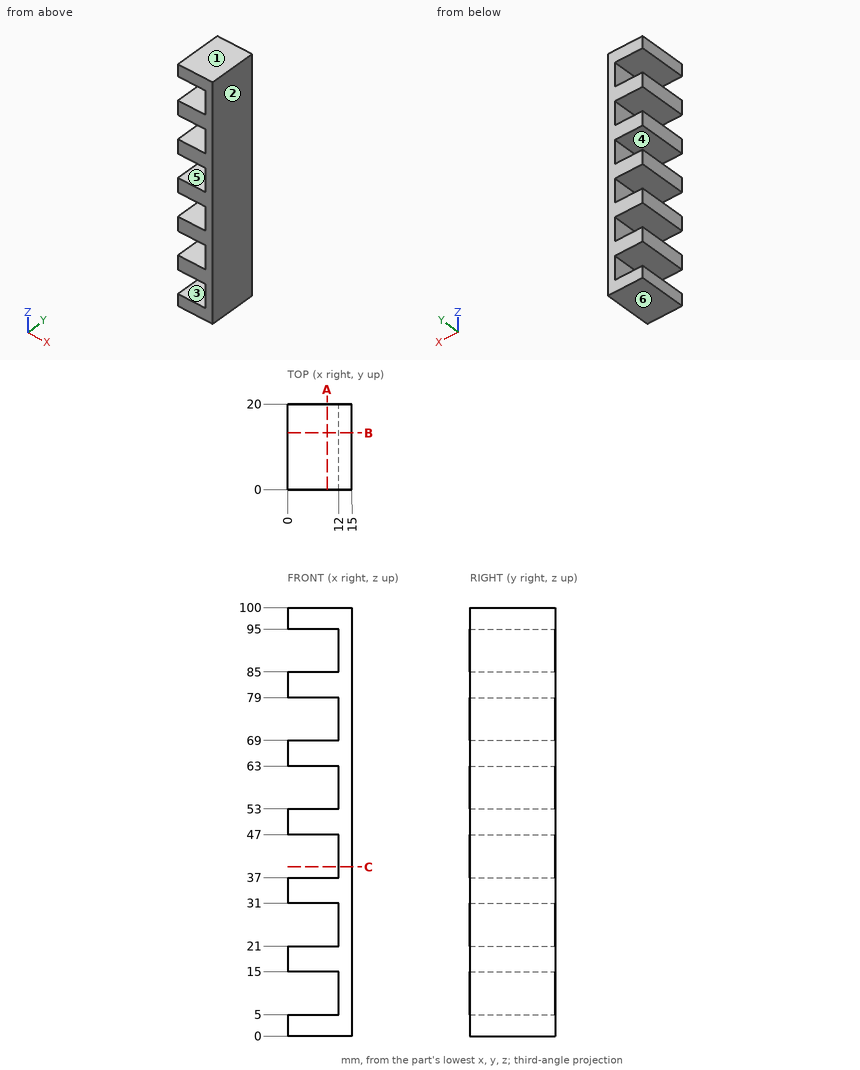
Verification items for this drawing (mm, ordinates from the low corner). A direction names the side the tool comes from. Give positions to 0.01 mm unless a question says otherwise; leave off trailing zeros. Loops run counter-clockwise (first coordinate to the right, second up) from the corner with the lowest first, then second, coordinate; pieces in that order, holes last.
1. Tool access check on the marked faces 5 and 6. Record the directions out of +Z, -Z, +X, -X, +Y, -Y that give a thin tool (end or side, any length) a straight path to the whole face; none if there is none.
Derived:
face 5: -X, +Y, -Y
face 6: -Z, +X, -X, +Y, -Y
2. Material ranges on probe 1 along X at (y, z) = (5, 9), recorded low to high.
Derived:
probe 1: x = 12 to 15
3. Release check for a two-part mould opening along Z. For the marked faces 1, 2, 3 and 4 record: +Z half, -Z half, draft (parallel to the pull), parting line (faces both ways), or undercut.
Derived:
face 1: +Z half
face 2: draft
face 3: undercut
face 4: undercut
4. Go/stop test with a flat-tipped pin: P1, Ø5, axis at y = 10.5, z = 44, coming from the -X side. Record where the tip stops, or that it passes through.
Derived:
P1: stops at x = 12
5. Cross-section at B-B on y = 13.25. Record the cut outline in (x, z), and give its area (3 significant figures).
Derived:
outline: (0, 0) - (15, 0) - (15, 100) - (0, 100) - (0, 95) - (12, 95) - (12, 85) - (0, 85) - (0, 79) - (12, 79) - (12, 69) - (0, 69) - (0, 63) - (12, 63) - (12, 53) - (0, 53) - (0, 47) - (12, 47) - (12, 37) - (0, 37) - (0, 31) - (12, 31) - (12, 21) - (0, 21) - (0, 15) - (12, 15) - (12, 5) - (0, 5) - close
area: 780 mm2
6. Cross-section at C-C on z = 39.5. Record the cut outline in (x, y).
Derived:
outline: (12, 0) - (15, 0) - (15, 20) - (12, 20) - close
7. Cross-section at A-A on x = 9.25. Record the cut outline in (y, z), and give its area (3 significant figures).
Derived:
outline: (0, 0) - (20, 0) - (20, 5) - (0, 5) - close; (0, 15) - (20, 15) - (20, 21) - (0, 21) - close; (0, 31) - (20, 31) - (20, 37) - (0, 37) - close; (0, 47) - (20, 47) - (20, 53) - (0, 53) - close; (0, 63) - (20, 63) - (20, 69) - (0, 69) - close; (0, 79) - (20, 79) - (20, 85) - (0, 85) - close; (0, 95) - (20, 95) - (20, 100) - (0, 100) - close
area: 800 mm2
